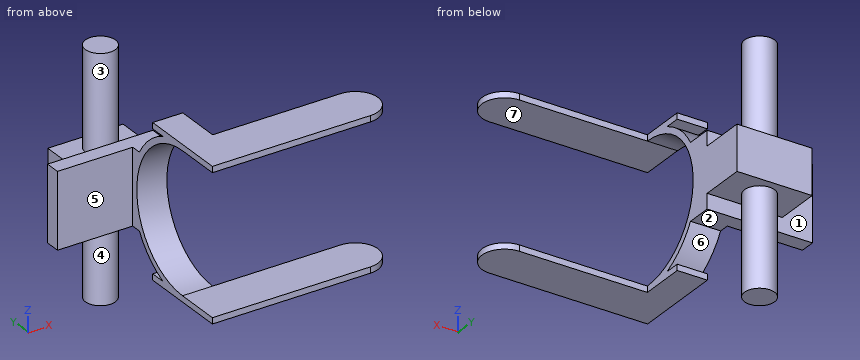
```python
from build123d import *

# Parameters (mm, degrees)
EXTRUDE_1_DEPTH     = 20
SKETCH_2_W          = 4
SKETCH_2_H          = 30
EXTRUDE_2_DEPTH     = 100
CUT_EXTRUDE_1_DEPTH = 100
SKETCH_4_W          = 50
SKETCH_4_H          = 10
EXTRUDE_3_DEPTH     = 50
SKETCH_5_W          = 50
SKETCH_5_H          = 30
EXTRUDE_4_DEPTH     = 30
SKETCH_6_R          = 10
EXTRUDE_5_DEPTH     = 80


with BuildPart() as part:
    # 草图1 → 凸台-拉伸1 (new body)
    with BuildSketch(Plane(origin=(0, 0, 0), x_dir=(0, 0, -1), z_dir=(1, 0, 0))):
        with BuildLine():
            Line((-25, 5), (25, 5))
            Line((25, 5), (25, -5))
            Line((25, -5), (25, -11.698777218))
            ThreePointArc((25, -11.698777218), (37.410642162, -21.801835726), (46, -35.304382227))
            Line((46, -35.304382227), (46, -25.083062159))
            Line((46, -25.083062159), (50, -25.083062159))
            Line((50, -25.083062159), (50, -85.083062159))
            Line((50, -85.083062159), (46, -85.083062159))
            Line((46, -85.083062159), (46, -55.083062159))
            ThreePointArc((46, -55.083062159), (0, -9.083062159), (-46, -55.083062159))
            Line((-46, -55.083062159), (-46, -85.083062159))
            Line((-46, -85.083062159), (-50, -85.083062159))
            Line((-50, -85.083062159), (-50, -25.083062159))
            Line((-50, -25.083062159), (-46, -25.083062159))
            Line((-46, -25.083062159), (-46, -35.304382227))
            ThreePointArc((-46, -35.304382227), (-37.410642162, -21.801835726), (-25, -11.698777218))
            Line((-25, -11.698777218), (-25, -5))
            Line((-25, -5), (-25, 5))
        make_face()
    extrude(amount=EXTRUDE_1_DEPTH)

    # 草图2 → 凸台-拉伸2 (add)
    with BuildSketch(Plane(origin=(20, 0, 0), x_dir=(0, 0, -1), z_dir=(1, 0, 0))):
        with Locations((-48, -70.083062159)):
            Rectangle(SKETCH_2_W, SKETCH_2_H)
        with Locations((48, -70.083062159)):
            Rectangle(SKETCH_2_W, SKETCH_2_H)
    extrude(amount=EXTRUDE_2_DEPTH)

    # 草图3 → 切除-拉伸1 (cut)
    with BuildSketch(Plane.XY.offset(50)):
        with BuildLine():
            Line((105, -55.083062159), (132.360099234, -55.083062159))
            Line((132.360099234, -55.083062159), (132.360099234, -85.083062159))
            Line((132.360099234, -85.083062159), (105, -85.083062159))
            ThreePointArc((105, -85.083062159), (120, -70.083062159), (105, -55.083062159))
        make_face()
    extrude(amount=-CUT_EXTRUDE_1_DEPTH, mode=Mode.SUBTRACT)

    # 草图4 → 凸台-拉伸3 (add)
    with BuildSketch(Plane.ZY):
        Rectangle(SKETCH_4_W, SKETCH_4_H)
    extrude(amount=EXTRUDE_3_DEPTH)

    # 草图5 → 凸台-拉伸4 (add)
    with BuildSketch(Plane(origin=(0, 5, 0), x_dir=(1, 0, 0), z_dir=(0, 1, 0))):
        with Locations((-5, 0)):
            Rectangle(SKETCH_5_W, SKETCH_5_H)
    extrude(amount=EXTRUDE_4_DEPTH)

    # 草图6 → 凸台-拉伸5 (add, symmetric)
    with BuildSketch(Plane.XY):
        with Locations((-5, 19.891808083)):
            Circle(SKETCH_6_R)
    extrude(amount=EXTRUDE_5_DEPTH, both=True)


solid = part.part
```
Verification items for the finished model (mm, model axes). Face numbers are marked on the shaded views. A direction names the side the tool comes from. Round coordinates to 2 decimals unless told otherwise and drop trailing zeros. Order: outer loops, then holes, each group sorted by start corner. A loop starts at its lowest first (then second) coordinate and runs counter-clockwise, first axis right, second up. Notation, with made-up numbers: (72, 51.25) -> (113, 51.25) arc R22 ccw to (113, 75.25) -> close; hole circle Ø8 at (-13.75, 73.5). An arc over 180 degrees is marked (long way). Put each result on its own line as item: value. Start each with the question number.
(1) Material ranges on line 1 along Z through (x, y) = (42, -70); line 2 along X through (y, z) = (-12, -23); line 3 along Y through (x, z) = (-39, -6.5), recorded low to high.
(2) Section check B-B (y = -29). Enter the section's corners in (x, z), then the cut area to 3 significant figures.
(3) Section check A-A (x = 48). Enter the section's corners in (y, z).
(4) Section check D-D (z = 0). Enter the section's corners in (x, y), then the cut area to 3 significant figures.
(5) Draft check along Y on the marked faces 5, 6 and 7. Enter one of: +Y half, -Y half, draft (parallel to the pull), parting line (faces both ways), or undercut.
(6) Section check C-C (x = -5). Enter the section's corners in (y, z), then the cut area to 3 significant figures.
(7) Depth check by flat-ended pin: pin 1 Ø1.5 at (y, z) = (15.5, 6.5) entering from -X; pin 2 Ø9 at (x, y) = (82.5, -76) entering from -Z; pin 3 Ø2 at (x, z) = (7, 47.5) entering from +Y; pin 4 Ø24 at (y, z) = (-31.5, -5) entering from -X. Enter the tip coordinate at first touch or a pass-through.
(8) Tool access check on the marked faces 1, 2, 3 and 4. Record the directions out of +Z, -Z, +X, -X, +Y, -Y that give a thin tool (end or side, any length) a straight path to the whole face; none if there is none.
Completed:
1. line 1: z = -50 to -46, 46 to 50
1. line 2: x = 0 to 20
1. line 3: y = -5 to 5
2. outline: (0, -50) -> (20, -50) -> (20, -46) -> (0, -46) -> close; (0, -42.74) -> (20, -42.74) -> (20, -37.89) -> (0, -37.89) -> close; (0, 37.89) -> (20, 37.89) -> (20, 42.74) -> (0, 42.74) -> close; (0, 46) -> (20, 46) -> (20, 50) -> (0, 50) -> close
2. area: 354 mm2
3. outline: (-85.08, -50) -> (-55.08, -50) -> (-55.08, -46) -> (-85.08, -46) -> close; (-85.08, 46) -> (-55.08, 46) -> (-55.08, 50) -> (-85.08, 50) -> close
4. outline: (-50, -5) -> (0, -5) -> (0, -9.08) -> (20, -9.08) -> (20, 35) -> (-30, 35) -> (-30, 5) -> (-50, 5) -> close
4. area: 2,280 mm2
5. face 5: -Y half
5. face 6: undercut
5. face 7: draft
6. outline: (-5, -25) -> (5, -25) -> (5, -15) -> (9.89, -15) -> (9.89, -80) -> (29.89, -80) -> (29.89, -15) -> (35, -15) -> (35, 15) -> (29.89, 15) -> (29.89, 80) -> (9.89, 80) -> (9.89, 15) -> (5, 15) -> (5, 25) -> (-5, 25) -> close
6. area: 4,000 mm2
7. pin 1: stops at x = -30
7. pin 2: stops at z = -50
7. pin 3: stops at y = -25.08
7. pin 4: passes through
8. face 1: -X
8. face 2: -Z, +X, -X
8. face 3: +Z
8. face 4: -Z
